Here's how the part is built. I have some questions about the finished solid (model axes, mm). Face numbers are marked on the shaded views. A direction names the side the tool comes from. Give positions to 0.01 mm unless a question says otherwise; leave off trailing zeros. Loops run counter-clockwise (first coordinate to the right, second up) from the corner with the lowest first, then second, coordinate; pieces in that order, holes last.
Q1. Will these pins go through, and if not, where does the flat tip stop? P1, Ø1.5, axis at x = 4.5, y = -423, coming from the +Z side; P2, Ø1, axis at x = 6.5, z = 409.5, coming from the +Y side; P3, Ø15, axis at y = -164, z = 13, coming from the +X side; P4, Ø2, axis at x = 0, y = -279, coming from the -Z side.
Q2. For the marked faces 1 and 2, which set-ups out of +Z, -Z, +X, -X, +Y, -Y let a thin tool reach every point of the face, with its end or its side?
Q3. If we section it at B-B (y = -270): Please give me the cut outline in (x, z), plus the area to 3 significant figures.
Q4. If we section it at A-A (x = 0): Please give me the cut outline in (y, z) (1 decimal), plus the area to 3 significant figures.
Q5. I need wall thicknesses on line 1 (Y direction, x = 0, z = 20.5) (1 decimal); line 2 (Y direction, x = 0, z = 59); line 3 (Z direction, x = -8, y = -205). Which ranges of each line are inside material? Lowest first, please.
from build123d import *

# Parameters (mm, degrees)
F1_DEPTH = 50.8
F2_R     = 12.8905
F3_DEPTH = 50.8
F0_R     = 12.8905


with BuildPart() as f1:
    # F0 (on Top) → F1 (new body)
    with BuildSketch(Plane.XY):
        with BuildLine():
            ThreePointArc((12.8905, -9.2655617612), (15.1104651235, -4.8671828351), (15.875, 0))
            ThreePointArc((15.875, 0), (-4.8671828351, 15.1104651235), (-12.8905, -9.2655617612))
            ThreePointArc((-12.8905, -9.2655617612), (0, -15.875), (12.8905, -9.2655617612))
        make_face()
        with BuildLine():
            ThreePointArc((12.8905, -9.2655617612), (0, -15.875), (-12.8905, -9.2655617612))
            Line((-12.8905, -9.2655617612), (-12.8905, -221.9905617612))
            Line((-12.8905, -221.9905617612), (12.8905, -221.9905617612))
            Line((12.8905, -221.9905617612), (12.8905, -9.2655617612))
        make_face()
        with BuildLine():
            Line((12.8905, -221.9905617612), (-12.8905, -221.9905617612))
            Line((-12.8905, -221.9905617612), (-12.8905, -434.7155617612))
            ThreePointArc((-12.8905, -434.7155617612), (0, -428.3226569569), (12.8905, -434.7155617612))
            Line((12.8905, -434.7155617612), (12.8905, -221.9905617612))
        make_face()
    extrude(amount=F1_DEPTH)

    # F2 (on face) → F3 (cut, through all)
    with BuildSketch(Plane.XY.offset(50.8)):
        Circle(F2_R)
    extrude(amount=-F3_DEPTH, mode=Mode.SUBTRACT)

    # F5: sweep along a path in F4
    with BuildLine(Plane.YZ) as f5_path:
        Line((-444.5151569569, 0), (-444.5151569569, 76.2))
        Line((-444.5151569569, 76.2), (-495.3151569569, 571.5))
        Line((-495.3151569569, 571.5), (-495.3151569569, 647.7))
    # F0 (on Top) → F5 (sweep)
    with BuildSketch(Plane.XY):
        with BuildLine():
            ThreePointArc((12.8905, -434.7155617612), (0, -428.3226569569), (-12.8905, -434.7155617612))
            ThreePointArc((-12.8905, -434.7155617612), (-5.1704755584, -459.8599684171), (16.1925, -444.5151569569))
            ThreePointArc((16.1925, -444.5151569569), (15.3448114602, -439.3446813985), (12.8905, -434.7155617612))
        make_face()
        with Locations((0, -444.5151569569)):
            Circle(F0_R, mode=Mode.SUBTRACT)
    sweep(path=f5_path.line, transition=Transition.RIGHT)


solid = f1.part
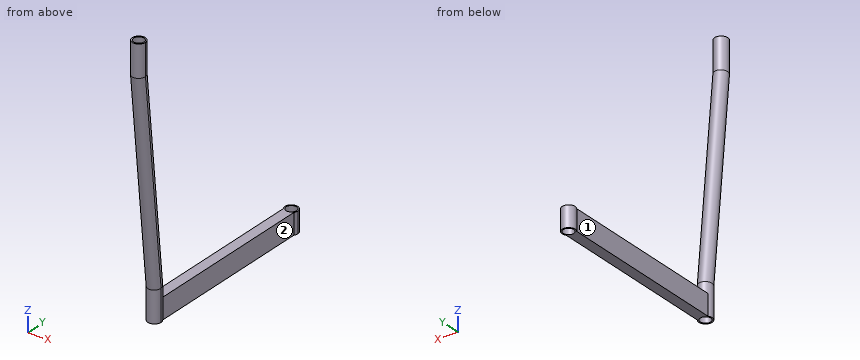
Check sheet entries:
1. P1: stops at z = 50.8
1. P2: stops at y = -463.57
1. P3: stops at x = 12.89
1. P4: stops at z = 0
2. face 1: +Z, -Z, -X
2. face 2: +Z, -Z, +X
3. outline: (-12.89, 0) - (12.89, 0) - (12.89, 50.8) - (-12.89, 50.8) - close
3. area: 1,310 mm2
4. outline: (-511.5, 570.7) - (-460.7, 75.4) - (-460.7, 0) - (-457.4, 0) - (-457.4, 75.5) - (-508.2, 570.8) - (-508.2, 647.7) - (-511.5, 647.7) - close; (-482.4, 572.2) - (-431.6, 76.9) - (-431.6, 0) - (-12.9, 0) - (-12.9, 50.8) - (-428.3, 50.8) - (-428.3, 77) - (-479.1, 572.3) - (-479.1, 647.7) - (-482.4, 647.7) - close; (12.9, 0) - (15.9, 0) - (15.9, 50.8) - (12.9, 50.8) - close
4. area: 25,600 mm2
5. line 1: y = -460.7 to -457.4, -431.6 to -12.9, 12.9 to 15.9
5. line 2: y = -460.71 to -457.41, -431.62 to -428.32
5. line 3: z = 0 to 50.8
